from build123d import *

# Parameters (mm, degrees)
BOSS_EXTRUDE1_DEPTH      = 14
BOSS_EXTRUDE1_DEPTH_BACK = 14
SKETCH1_R                = 38
SKETCH1_R_2              = 35
BOSS_EXTRUDE2_DEPTH      = 5
BOSS_EXTRUDE2_DEPTH_BACK = 5
SKETCH2_R                = 35
SKETCH5_R                = 20
SKETCH5_R_2              = 15
BOSS_EXTRUDE3_DEPTH      = 15
BOSS_EXTRUDE4_START      = 15
SKETCH6_R                = 20
SKETCH6_R_2              = 15
BOSS_EXTRUDE4_DEPTH      = 15
DRAFT2_ANGLE             = 35
DRAFT3_ANGLE             = 35
SKETCH14_R               = 12
CUT_EXTRUDE3_DEPTH       = 15
SKETCH15_R               = 15
CUT_EXTRUDE4_DEPTH       = 33.5


with BuildPart() as part:
    # Sketch1 → Boss-Extrude1 (new, two sides: drawn at the far end of the back side and taken through both)
    with BuildSketch(Plane(origin=(0, 0, 0), x_dir=(1, 0, 0), z_dir=(0, 1, 0)).offset(-BOSS_EXTRUDE1_DEPTH_BACK)):
        with Locations(Location((0, 0, 0), (0, 0, 270))):
            Circle(SKETCH1_R)
        with Locations(Location((0, 0, 0), (0, 0, 270))):
            Circle(SKETCH1_R_2, mode=Mode.SUBTRACT)
    extrude(amount=BOSS_EXTRUDE1_DEPTH + BOSS_EXTRUDE1_DEPTH_BACK)

    # Sketch2 → Boss-Extrude2 (add, two sides: drawn at the far end of the back side and taken through both)
    with BuildSketch(Plane(origin=(0, 0, 0), x_dir=(-1, 0, 0), z_dir=(0, -1, 0)).offset(-BOSS_EXTRUDE2_DEPTH_BACK)):
        with Locations(Location((0, 0, 0), (0, 0, 270))):
            Circle(SKETCH2_R)
    extrude(amount=BOSS_EXTRUDE2_DEPTH + BOSS_EXTRUDE2_DEPTH_BACK)

    # Sketch5 → Boss-Extrude3 (add)
    with BuildSketch(Plane(origin=(0, 5, 0), x_dir=(1, 0, 0), z_dir=(0, 1, 0))):
        Circle(SKETCH5_R)
        with Locations(Location((0, 0, 0), (0, 0, 180))):
            Circle(SKETCH5_R_2, mode=Mode.SUBTRACT)
    extrude(amount=BOSS_EXTRUDE3_DEPTH)

    # Sketch6 → Boss-Extrude4 (add)
    with BuildSketch(Plane.XZ.offset(5).offset(BOSS_EXTRUDE4_START)):
        Circle(SKETCH6_R)
        with Locations(Location((0, 0, 0), (0, 0, 180))):
            Circle(SKETCH6_R_2, mode=Mode.SUBTRACT)
    extrude(amount=-BOSS_EXTRUDE4_DEPTH)

    # Draft2
    draft2_faces = [part.faces().sort_by_distance(p)[0] for p in [
        (-20, 12.5, 0),
    ]]
    draft(draft2_faces, Plane(origin=(0, 20, 0), x_dir=(1, 0, 0), z_dir=(0, 1, 0)), DRAFT2_ANGLE)

    # Draft3
    draft3_faces = [part.faces().sort_by_distance(p)[0] for p in [
        (-20, -12.5, 0),
    ]]
    draft(draft3_faces, Plane(origin=(0, -20, 0), x_dir=(-1, 0, 0), z_dir=(0, -1, 0)), DRAFT3_ANGLE)

    # Sketch14 → Cut-Extrude3 (cut)
    with BuildSketch(Plane.XZ.offset(5)):
        Circle(SKETCH14_R)
    extrude(amount=-CUT_EXTRUDE3_DEPTH, mode=Mode.SUBTRACT)

    # Sketch15 → Cut-Extrude4 (cut, symmetric)
    with BuildSketch(Plane(origin=(0, 5, 0), x_dir=(1, 0, 0), z_dir=(0, 1, 0))):
        Circle(SKETCH15_R)
    extrude(amount=CUT_EXTRUDE4_DEPTH, both=True, mode=Mode.SUBTRACT)


solid = part.part
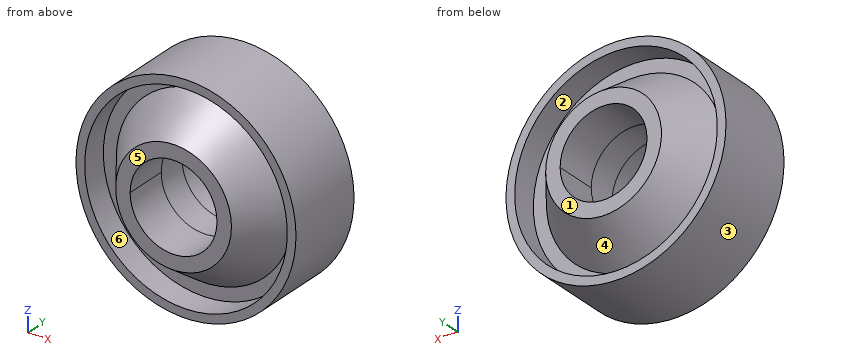
Verification items for the finished model (mm, model axes). Face numbers are marked on the shaded views. A direction names the side the tool comes from. Give positions to 0.01 mm unless a question says otherwise; leave off trailing zeros. Write each loop counter-clockwise with the first axis right and the second up, starting at its lowest first coordinate (ties: lowest second). Pieces come first, ordered by that corner, then holes. Notation, with made-up numbers: M 51,17.5 L 109,17.5 A29 ccw 109,53.5 Z; hole C 60,28.5 d10. An arc over 180 degrees is marked long. Use CSV: the item, a comma, the result in double quotes.
1) Release check for a two-part mould opening along X. For the marked faces 1, 2, 3 and 4 record: released by +X, released by -X, zero draft, split by the parting line, or undercut.
Final values:
face 1,"zero draft"
face 2,"undercut"
face 3,"split by the parting line"
face 4,"undercut"
2) Cross-section at B-B (y = -13). Enter the section's corners in (x, z).
Final values:
outline,"C 0,0 d76; C 0,0 d49.8; hole C 0,0 d70; hole C 0,0 d30"
3) Cross-section at D-D (x = 31.5). Enter the section's corners in (y, z).
Final values:
outline,"M -14,-21.25 L 14,-21.25 L 14,-15.26 L 5,-15.26 L 5,15.26 L 14,15.26 L 14,21.25 L -14,21.25 L -14,15.26 L -5,15.26 L -5,-15.26 L -14,-15.26 Z"
4) Cross-section at C-C (y = 0). Enter the section's corners in (x, z).
Final values:
outline,"C 0,0 d76; hole C 0,0 d30"
5) Material ranges on line 1 along X through (y, z) = (0.5, -0.5); line 2 along Z through (x, y) = (-5, -2); line 3 along Y through (x, z) = (33, 9), recorded low to high.
Final values:
line 1,"-38 to -14.99, 14.99 to 38"
line 2,"-37.67 to -14.14, 14.14 to 37.67"
line 3,"-5 to 5"
6) Cross-section at A-A (x = 0). Enter the section's corners in (y, z).
Final values:
outline,"M -20,-20 L -5,-30.5 L -5,-35 L -14,-35 L -14,-38 L 14,-38 L 14,-35 L 5,-35 L 5,-30.5 L 20,-20 L 20,-15 L -20,-15 Z; M -20,15 L 20,15 L 20,20 L 5,30.5 L 5,35 L 14,35 L 14,38 L -14,38 L -14,35 L -5,35 L -5,30.5 L -20,20 Z"
7) Go/stop test with flat-tipped pins: pin 1 Ø8 at (y, z) = (2, 19) entering from -X; pin 2 Ø12 at (y, z) = (-10, -28.5) entering from +X; pin 3 Ø5 at (y, z) = (1, -3.5) entering from -X. Record where each tip stops, or that it passes through.
Final values:
pin 1,"x = -34.91"
pin 2,"x = 30.62"
pin 3,"x = -37.99"
8) Access from +Z, -Z, +X, -X, +Y, -Y to the whole of each face (thin tool, end or side, straight path). Record for the marked faces 5 and 6.
Final values:
face 5,"+Z, -Z, +X, -X, -Y"
face 6,"-Y"
